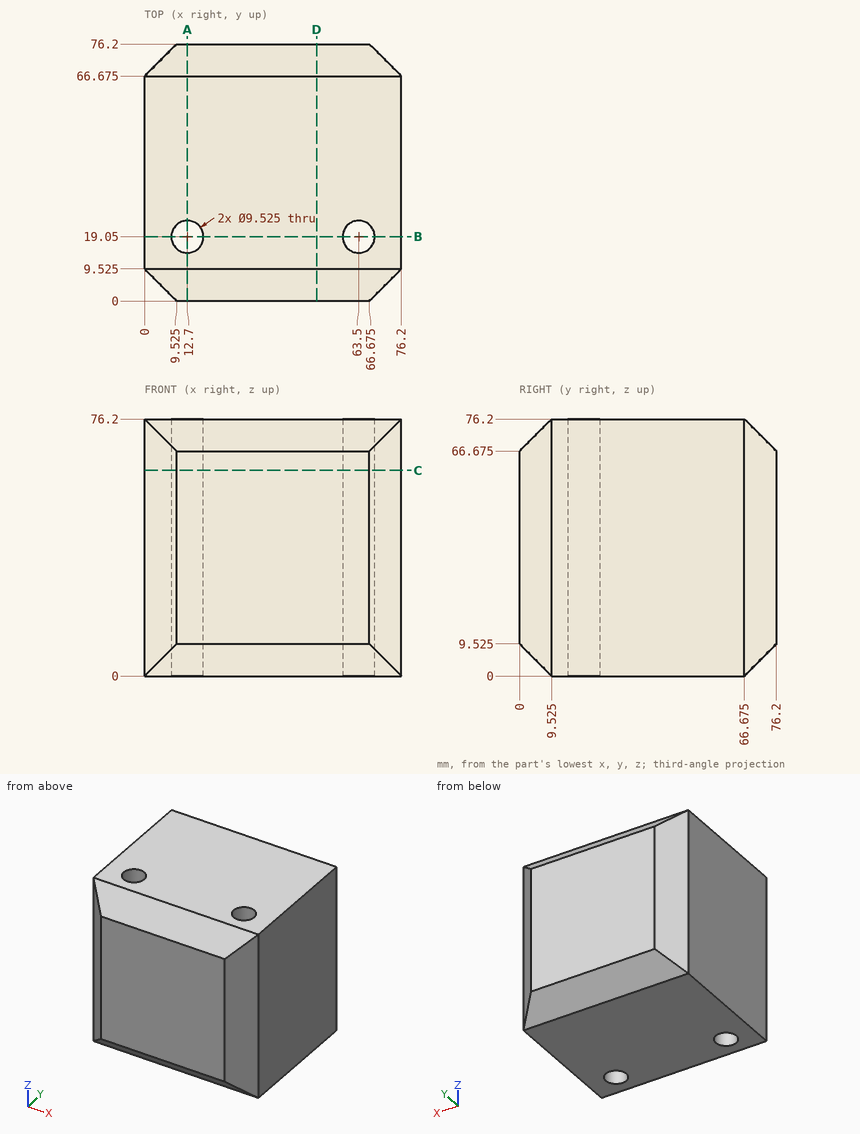
Geometry check sheet. Reference: drawing and pictorial views, mm from the part's lowest x, y, z. Give positions to 0.01 mm unless a question says otherwise; leave off trailing zeros. Order: outer loops, then holes, each group sorted by start corner. A loop starts at its lowest first (then second) coordinate and runs counter-clockwise, first axis right, second up. Notation, with made-up numbers: (-40, 63) -> (-22, 63) arc R28 cw to (-22, 99) -> close; hole circle Ø1 at (2, 58). An arc over 180 degrees is marked (long way). Use CSV: the item, a comma, the result in double quotes. Start each with the question number.
1) Sectioned sample at D-D, the plane x = 51. Record the boundary of the cut face in (y, z) (3 decimals).
2) Sectioned sample at A-A, the plane x = 12.7. Record the boundary of the cut face in (y, z) (1 decimal).
3) Sectioned sample at B-B, the plane y = 19.05. Record the boundary of the cut face in (x, z).
4) Material ranges on line 1 (X direction, y = 19, z = 32); line 2 (Y direction, x = 63.5, z = 19); line 3 (Y direction, x = 64, z = 7) (3 decimals), recorded low to high. Write a range as from..to.
5) Go/stop test with flat-tipped pins: P1, Ø8.5, axis at x = 63.5, y = 19.05, coming from the -Z side; P2, Ø1.5, axis at y = 8.5, z = 42, coming from the -X side (3 decimals); P3, Ø1, axis at x = 21, z = 67, coming from the +Y side. Record where each tip stops, or that it passes through.
6) Sectioned sample at C-C, the plane z = 61. Give the number of separate pieces and of enclosed holes in the cut face, plus the area to 3 significant figures.
Recorded:
1,outline,"(0, 9.525) -> (9.525, 0) -> (66.675, 0) -> (76.2, 9.525) -> (76.2, 66.675) -> (66.675, 76.2) -> (9.525, 76.2) -> (0, 66.675) -> close"
2,outline,"(0, 9.5) -> (9.5, 0) -> (14.3, 0) -> (14.3, 76.2) -> (9.5, 76.2) -> (0, 66.7) -> close; (23.8, 0) -> (66.7, 0) -> (76.2, 9.5) -> (76.2, 66.7) -> (66.7, 76.2) -> (23.8, 76.2) -> close"
3,outline,"(0, 0) -> (7.94, 0) -> (7.94, 76.2) -> (0, 76.2) -> close; (17.46, 0) -> (58.74, 0) -> (58.74, 76.2) -> (17.46, 76.2) -> close; (68.26, 0) -> (76.2, 0) -> (76.2, 76.2) -> (68.26, 76.2) -> close"
4,line 1,"0..7.94, 17.46..58.74, 68.26..76.2"
4,line 2,"0..14.29, 23.81..76.2"
4,line 3,"2.525..14.314, 23.786..73.675"
5,P1,"through"
5,P2,"x = 0.275"
5,P3,"y = 76.2"
6,separate pieces,"1"
6,enclosed holes,"2"
6,area,"5,480 mm2"
